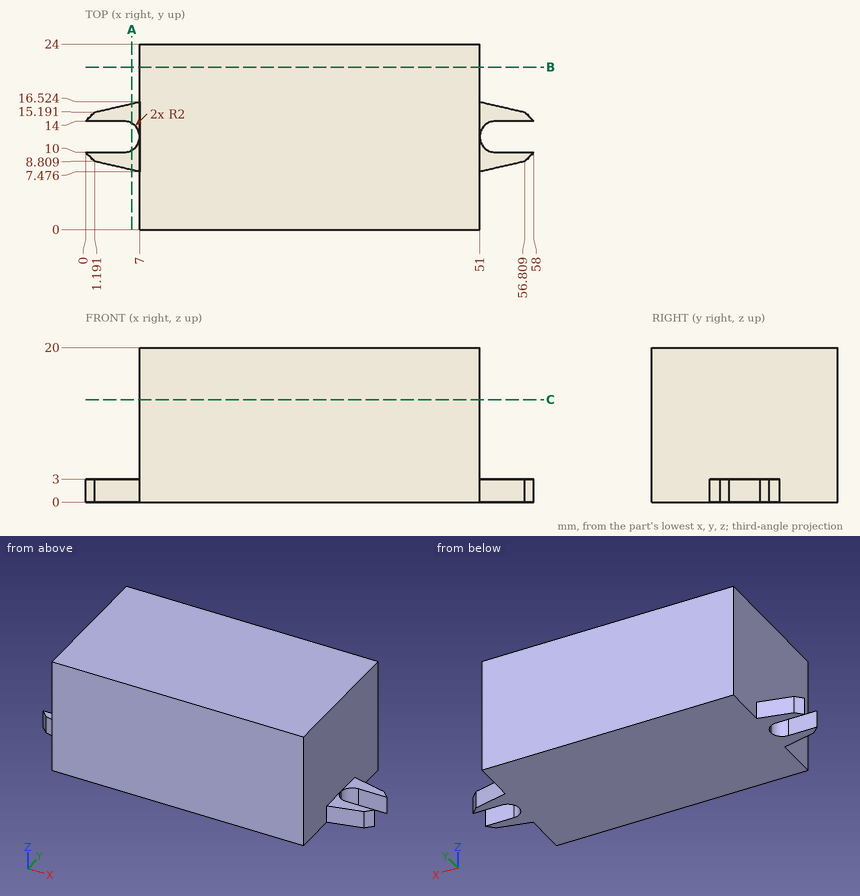
Here's the drawing with two shaded views (mm, measured from the low corner). I have some questions. Coordinates: 2 decimals unless noted, no trailing zeros. Loops run counter-clockwise (first coordinate to the right, second up) from the corner with the lowest first, then second, coordinate; pieces in that order, holes last. Notation, with made-up numbers: (1.5, 22) -> (20.5, 22) arc R22 cw to (20.5, 45) -> close; hole circle Ø2 at (6.5, 31). An arc over 180 degrees is marked (long way). Answer as a JSON object with one key per item and string values.
1) Imagine slicing it at B-B (y = 21). Please give me the cut outline in (x, z), then the cut area to 3 significant figures.
Results:
{"outline": "(7, 0) -> (51, 0) -> (51, 20) -> (7, 20) -> close", "area": "880 mm^2"}
2) For P1, Ø3, axis at y = 2.5, z = 11, coming from the -X side; P2, Ø1, axis at y = 19, z = 9.5, coming from the +X side; P3, Ø3.5, axis at x = 54.5, z = 1, coming from the +Y side; P4, Ø4, axis at x = 46.5, z = 11.5, coming from the -Y side, each with a flat end and sliding along its axis, tell me the tip position at first contact or that it passes through.
Results:
{"P1": "stops at x = 7", "P2": "stops at x = 51", "P3": "stops at y = 16.12", "P4": "stops at y = 0"}
3) If I drill on line 1 (X direction, y = 17.75, z = 16.5), over which ranges is the centre line in solid material (lowest first)?
Results:
{"line 1": "x = 7 to 51"}
4) Imagine slicing it at C-C (z = 13.25). Please give me the cut outline in (x, y).
Results:
{"outline": "(7, 0) -> (51, 0) -> (51, 24) -> (7, 24) -> close"}
5) Imagine slicing it at A-A (x = 6). Please give me the cut outline in (y, z).
Results:
{"outline": "(7.71, 0) -> (10.27, 0) -> (10.27, 3) -> (7.71, 3) -> close; (13.73, 0) -> (16.29, 0) -> (16.29, 3) -> (13.73, 3) -> close"}
